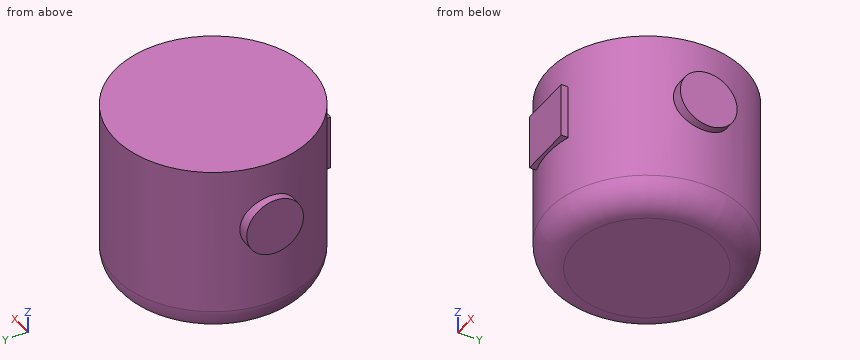
from build123d import *

# Parameters (mm, degrees)
F0_R     = 56.608294
F1_DEPTH = 101.6
F2_R     = 15.24
F3_W     = 31.386364
F3_H     = 31.386374
F4_DEPTH = 58.42
F5_R     = 16.335197
F6_DEPTH = 60.96


with BuildPart() as f1:
    # F0 (on Top) → F1 (new body)
    with BuildSketch(Plane.XY):
        Circle(F0_R)
    extrude(amount=F1_DEPTH)

    # F2
    f2_edges = [f1.edges().sort_by_distance(p)[0] for p in [
        (-56.608294, 0, 0),
    ]]
    fillet(f2_edges, radius=F2_R)

    # F3 (on Front) → F4 (join)
    with BuildSketch(Plane.XZ):
        with Locations((0, 65.980129)):
            Rectangle(F3_W, F3_H)
    extrude(amount=F4_DEPTH)

    # F5 (on Right) → F6 (join, symmetric)
    with BuildSketch(Plane.YZ):
        with Locations((0, 65.102533)):
            Circle(F5_R)
    extrude(amount=F6_DEPTH, both=True)


solid = f1.part
Geometry check sheet. Reference: the model listing, model coordinates, mm. Round coordinates to 2 decimals unless told otherwise and drop trailing zeros. Order: outer loops, then holes, each group sorted by start corner. A loop starts at its lowest first (then second) coordinate and runs counter-clockwise, first axis right, second up. Notation, with made-up numbers: M -12.75,-34.5 L 43.25,-34.5 A31 cw 43.25,4.5 Z; hole C 37,-10.5 d8. An arc over 180 degrees is marked long. Write each question's results on one line, items separated by ' | '. Start each with the question number.
1. Material ranges on L1, parallel to X at y = -20.5, z = 83; L2, parallel to Y at x = -39.5, z = 64; L3, parallel to Y at x = 9.5, z = 72, recorded low to high. Write a range as from..to.
2. Cross-section at D-D on z = 31.5. Record the boundary of the cut face in (x, y).
3. Cross-section at B-B on x = 0. Record the boundary of the cut face in (y, z).
4. Cross-section at A-A on y = 0. Record the boundary of the cut face in (x, z).
5. Go/stop test with flat-tipped pins: P1, Ø2, axis at x = 1, z = 29, coming from the -Y side; P2, Ø2, axis at y = 8, z = 13, coming from the +X side; P3, Ø2, axis at y = -57, z = 64.5, coming from the -X side; P4, Ø3, axis at x = 8, y = -57.5, coming from the +Z side. Record where each tip stops, or that it passes through.
6. Cross-section at C-C on z = 59.5. Record the boundary of the cut face in (x, y).
Resolved:
1) L1: -52.77..52.77 | L2: -40.55..40.55 | L3: -58.42..55.81
2) outline: C 0,0 d113.22
3) outline: M -58.42,50.29 L -56.61,50.29 L -56.61,15.24 A15.24 ccw -41.37,0 L 41.37,0 A15.24 ccw 56.61,15.24 L 56.61,101.6 L -56.61,101.6 L -56.61,81.67 L -58.42,81.67 Z
4) outline: M -60.96,48.77 L -56.61,48.77 L -56.61,15.24 A15.24 ccw -41.37,0 L 41.37,0 A15.24 ccw 56.61,15.24 L 56.61,48.77 L 60.96,48.77 L 60.96,81.44 L 56.61,81.44 L 56.61,101.6 L -56.61,101.6 L -56.61,81.44 L -60.96,81.44 Z
5) P1: y = -56.61 | P2: x = 56.06 | P3: x = -15.69 | P4: z = 101.6
6) outline: M -60.96,-15.34 L -54.49,-15.34 A56.61 ccw -15.69,-54.39 L -15.69,-58.42 L 15.69,-58.42 L 15.69,-54.39 A56.61 ccw 54.49,-15.34 L 60.96,-15.34 L 60.96,15.34 L 54.49,15.34 A56.61 ccw -54.49,15.34 L -60.96,15.34 Z
